Model file for the job. Use its own axes, mm. Coordinates: 2 decimals unless noted, no trailing zeros. Order: outer loops, then holes, each group sorted by start corner. A loop starts at its lowest first (then second) coordinate and runs counter-clockwise, first axis right, second up. Notation, with made-up numbers: M -39.75,-30.5 L -4.75,-30.5 A6 ccw -4.75,-23.5 Z; hole C -14.5,64 d3. An arc over 180 degrees is marked long. Return JSON: item names as keys, results as strings.
Autodesk Inventor part; units mm, degrees
ref_plane "YZ Plane" through (0, 0, 0) normal (1, 0, 0) x (0, 1, 0)
ref_plane "XY Plane" through (0, 0, 0) normal (0, 0, 1) x (1, 0, 0)
ref_plane "工作平面1" through (0, 0, 1.5) normal (0, 0, -1) x (-1, 0, 0)
sketch "草圖1" plane through (0, 0, 0) normal (0, 0, 1) x (1, 0, 0)
  line L0 (0, 6) -> (0, -6)
  line L1 (0, -6) -> (-139, -6)
  line L2 (-139, -6) -> (-139, 6)
  line L3 (-149, 2) -> (-139, 2)
  line L4 (-139, 2) -> (-139, -2)
  line L5 (-139, -2) -> (-149, -2)
  line L6 (-149, -2) -> (-149, 2)
  line L7 (0, -9.6) -> (0, 15.6)
  line L8 (-148, -2) -> (-139, -2)
  line L9 (-139, -2) -> (-139, -6)
  line L10 (-139, 6) -> (-139, 2)
  line L11 (-139, 2) -> (-148, 2)
  line L12 (-139, 6) -> (0, 6)
  line L13 (139, -6) -> (139, 6)
  line L14 (139, 6) -> (139, 2)
  line L15 (139, -2) -> (139, -6)
  line L16 (139, 2) -> (148, 2)
  line L17 (149, 2) -> (139, 2)
  line L18 (148, -2) -> (139, -2)
  line L19 (139, -2) -> (149, -2)
  line L20 (149, -2) -> (149, 2)
  line L21 (139, 2) -> (139, -2)
  line L22 (0, -6) -> (139, -6)
  line L23 (139, 6) -> (0, 6)
  point P0 (0, 0)
  point P1 (0, 0)
  point P2 (0, 0)
  dimension "d0" = 10
  dimension "d1" = 139
  dimension "d2" = 4
extrude "擠出1" add sketch "草圖1" along normal blind 3
ref_plane "工作平面1" through (0, 0, 1.5) normal (0, 0, -1) x (-1, 0, 0)
properties part number "rod_3"
Item 1: Wall check: line 1 (X direction, y = 2.25, z = 1.6). Give the ranges that are in metal, low to high.
Check result:
{"line 1": "x = -139 to 139"}
Item 2: Drop flat-ended pins along their axis: pin 1 Ø0.9 at (x, z) = (145, 1.5) entering from -Y; pin 2 Ø1.5 at (y, z) = (5, 1.5) entering from -X. Give the stop position or say it passes through.
Check result:
{"pin 1": "stops at y = -2", "pin 2": "stops at x = -139"}
Item 3: Saw through at B-B (y = -4). Write the cut outline in (x, z), and give its area (3 significant figures).
Check result:
{"outline": "M -139,0 L 139,0 L 139,3 L -139,3 Z", "area": "834 mm2"}
Item 4: Saw through at A-A (z = 1.35). Write the cut outline in (x, y), and give its area (3 significant figures).
Check result:
{"outline": "M -149,-2 L -139,-2 L -139,-6 L 139,-6 L 139,-2 L 149,-2 L 149,2 L 139,2 L 139,6 L -139,6 L -139,2 L -149,2 Z", "area": "3,420 mm2"}
